Here's the drawing with two shaded views (mm, measured from the low corner). I have some questions. Round coordinates to 2 decimals unless told otherwise and drop trailing zeros. Write each loop counter-clockwise with the first axis right and the second up, starting at its lowest first coordinate (ties: lowest second). Pieces come first, ordered by that corner, then holes. Notation, with made-up numbers: M 8.25,-26 L 35.25,-26 A8 cw 35.25,-12 Z; hole C -6,79.5 d11. An arc over 180 degrees is marked long. Use one line per item in the form item = value. Start each with the question number.
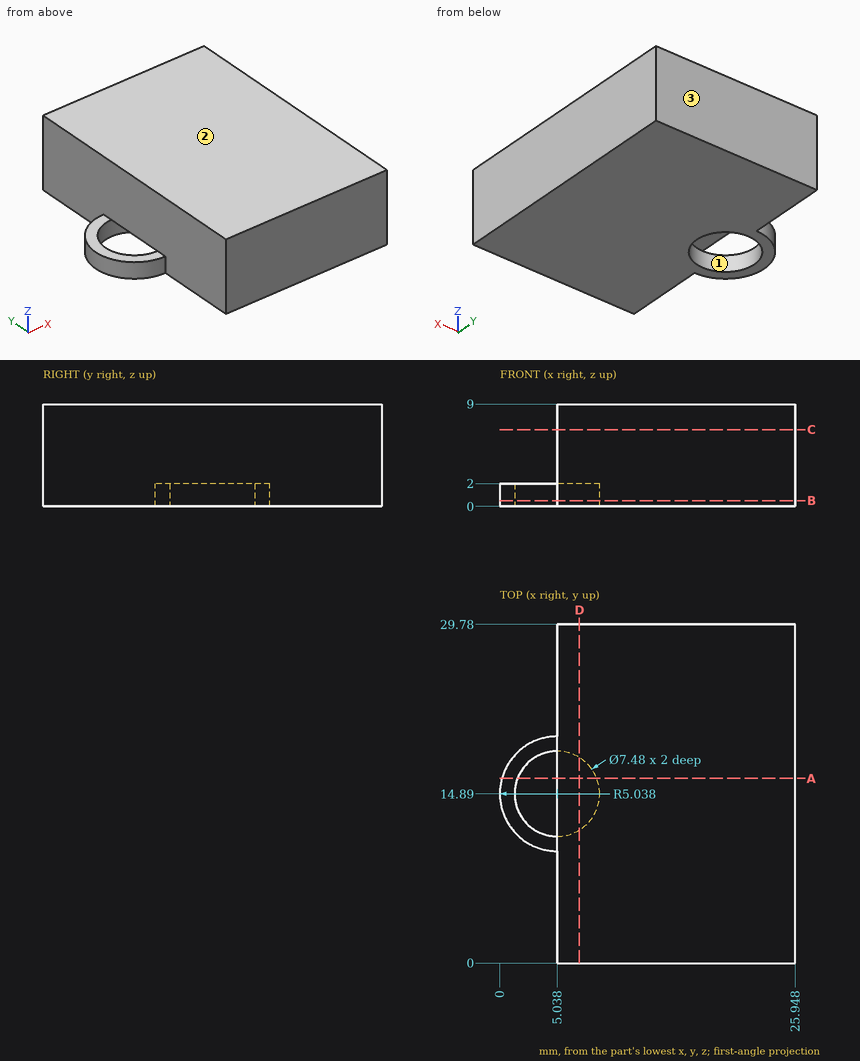
1. Will this pin go through, and if not, where does the flat tip stop? pin 1 (2 mm diameter, centred on y = 22, z = 2, fed in from -X).
2. If we section it at C-C (z = 6.75): List the corners of the cut face in (x, y) for me.
3. If we mould it in two halves opening along Y, with no side actions, what happens to the marked faces 1, 2 and 3? For each: pulls with the +Y half, pulls with the -Y half, needs draft (parallel to the pull), parting line crosses it, or undercut.
4. Please list where this line runs through material, in increasing order: line 1 along X through (y, z) = (17.75, 7.5).
5. If we section it at B-B (z = 0.5): List the corners of the cut face in (x, y) for me.
6. If we section it at A-A (y = 16.25): List the corners of the cut face in (x, z) for me.
7. If we section it at D-D (x = 7): List the corners of the cut face in (y, z) for me (1 decimal).
Model answer:
q1.pin_1 = 5.04
q2.outline = M 5.04,0 L 25.95,0 L 25.95,29.78 L 5.04,29.78 Z
q3.face_1 = undercut
q3.face_2 = needs draft
q3.face_3 = pulls with the +Y half
q4.line_1 = 5.04 to 25.95
q5.outline = M 5.04,0 L 25.95,0 L 25.95,29.78 L 5.04,29.78 L 5.04,19.93 A5.04 ccw 5.04,9.85 Z; hole C 5.04,14.89 d7.48
q6.outline = M 0.19,0 L 1.55,0 L 1.55,2 L 0.19,2 Z; M 5.04,2 L 8.52,2 L 8.52,0 L 25.95,0 L 25.95,9 L 5.04,9 Z
q7.outline = M 0,0 L 11.7,0 L 11.7,2 L 18.1,2 L 18.1,0 L 29.8,0 L 29.8,9 L 0,9 Z
